The model under review builds one solid part; all positions refer to its coordinate system, in mm. Face numbers are marked on the shaded views. A direction names the side the tool comes from. Round coordinates to 2 decimals unless told otherwise and drop trailing zeros. Order: outer loops, then holes, each group sorted by start corner. A loop starts at its lowest first (then second) coordinate and runs counter-clockwise, first axis right, second up.
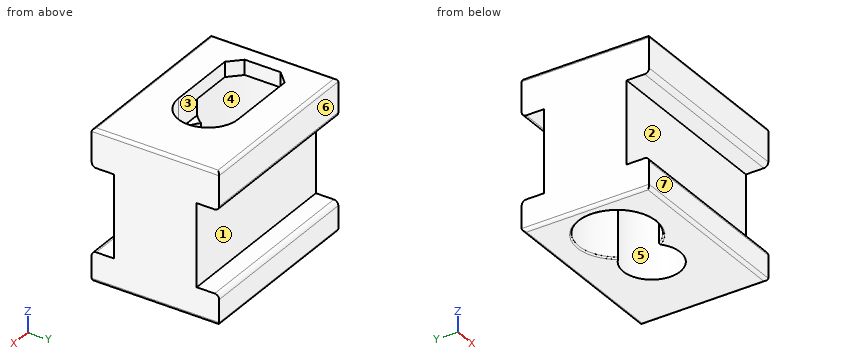
from build123d import *

# Parameters (mm, degrees)
ESQUISSE1_W             = 120
ESQUISSE1_H             = 85.2
BOSS_EXTRU_1_DEPTH      = 100
ESQUISSE2_W             = 55
ESQUISSE2_H             = 15
ENL_V_MAT_EXTRU_1_DEPTH = 121
CONG_1_R                = 3
CONG_2_R                = 2
CONG_3_R                = 2
ESQUISSE3_R             = 25.5
ENL_V_MAT_EXTRU_2_DEPTH = 90
CONG_4_R                = 1
ENL_V_MAT_EXTRU_3_DEPTH = 20.7
ESQUISSE6_R             = 19
ENL_V_MAT_EXTRU_5_DEPTH = 85


with BuildPart() as part:
    # Esquisse1 → Boss.-Extru.1 (new body)
    with BuildSketch(Plane.XY):
        Rectangle(ESQUISSE1_W, ESQUISSE1_H)
    extrude(amount=BOSS_EXTRU_1_DEPTH)

    # Esquisse2 → Enlèv. mat.-Extru.1 (cut, through all)
    with BuildSketch(Plane.ZY.offset(60)):
        with Locations((47.5, 35.1)):
            Rectangle(ESQUISSE2_W, ESQUISSE2_H)
        with Locations((47.5, -35.1)):
            Rectangle(ESQUISSE2_W, ESQUISSE2_H)
    extrude(amount=-ENL_V_MAT_EXTRU_1_DEPTH, mode=Mode.SUBTRACT)

    # Congé1
    cong_1_edges = [part.edges().sort_by_distance(p)[0] for p in [
        (0, 42.6, 75),
        (0, 42.6, 20),
        (0, -42.6, 20),
        (0, -42.6, 75),
    ]]
    fillet(cong_1_edges, radius=CONG_1_R)

    # Congé2
    cong_2_edges = [part.edges().sort_by_distance(p)[0] for p in [
        (0, -42.6, 0),
        (-60, 0, 0),
        (0, 42.6, 0),
        (60, 0, 0),
    ]]
    fillet(cong_2_edges, radius=CONG_2_R)

    # Congé3
    cong_3_edges = [part.edges().sort_by_distance(p)[0] for p in [
        (-60, 0, 100),
        (0, -42.6, 100),
        (60, 0, 100),
        (0, 42.6, 100),
    ]]
    fillet(cong_3_edges, radius=CONG_3_R)

    # Esquisse3 → Enlèv. mat.-Extru.2 (cut)
    with BuildSketch(Plane(origin=(0, 0, 0), x_dir=(-1, 0, 0), z_dir=(0, 0, -1))):
        with Locations((28, 0)):
            Circle(ESQUISSE3_R)
    extrude(amount=-ENL_V_MAT_EXTRU_2_DEPTH, mode=Mode.SUBTRACT)

    # Congé4
    cong_4_edges = [part.edges().sort_by_distance(p)[0] for p in [
        (-2.5, 0, 0),
    ]]
    fillet(cong_4_edges, radius=CONG_4_R)

    # Esquisse5 → Enlèv. mat.-Extru.3 (cut)
    with BuildSketch(Plane.XY.offset(100)):
        with BuildLine():
            Line((-48, 0), (-48, 12))
            Line((-48, 12), (-40, 20))
            Line((-40, 20), (-28, 20))
            Line((-28, 20), (6.8, 20))
            ThreePointArc((6.8, 20), (26.8, 0), (6.8, -20))
            Line((6.8, -20), (-28, -20))
            Line((-28, -20), (-40, -20))
            Line((-40, -20), (-48, -12))
            Line((-48, -12), (-48, 0))
        make_face()
    extrude(amount=-ENL_V_MAT_EXTRU_3_DEPTH, mode=Mode.SUBTRACT)

    # Esquisse6 → Enlèv. mat.-Extru.5 (cut)
    with BuildSketch(Plane.XY.offset(79.3)):
        with Locations((6.8, 0)):
            Circle(ESQUISSE6_R)
    extrude(amount=-ENL_V_MAT_EXTRU_5_DEPTH, mode=Mode.SUBTRACT)


solid = part.part
(1) To check wall thickness, follow L1, parallel to Y at x = -27, z = 5; L2, parallel to X at y = 0, z = 57; L3, parallel to Y at x = -11, z = 22. State the ranges of each line that lie inside material, in increasing order.
(2) We need section A-A (y = 34). Give the boundary of the cut face in (x, z).
(3) Tool access review of the marked faces 1, 2, 3 and 4: name each direction out of +Z, -Z, +X, -X, +Y, -Y from which nothing blocks a thin tool from reaching the whole face with its end or side.
(4) Clearance check with flat-ended pins moving along their axes: P1, Ø6, axis at x = 23, y = 9, coming from the +Z side; P2, Ø4, axis at x = 18, z = 23.5, coming from the -Y side; P3, Ø16.5, axis at x = -23, z = 60.5, coming from the +Y side. State where each tip first meets the part, or that it passes through.
(5) We need section B-B (z = 83). Give the boundary of the cut face in (x, y).
(6) The part is to be moulded in two halves that separate along Y. For the marked faces 5, 6 and 7, say which applies: pulls with the +Y half, pulls with the -Y half, needs draft (parallel to the pull), parting line crosses it, or undercut.
(7) We need section D-D (y = 0). Give the boundary of the cut face in (x, z).
Verdict:
1. L1: y = -42.6 to -25.48, 25.48 to 42.6
1. L2: x = -60 to -53.5, 25.8 to 60
1. L3: y = -27.6 to -19.01, 19.01 to 27.6
2. outline: (-60, 2) arc R2 ccw to (-58, 0) - (58, 0) arc R2 ccw to (60, 2) - (60, 20) - (-60, 20) - close; (-60, 75) - (60, 75) - (60, 98) arc R2 ccw to (58, 100) - (-58, 100) arc R2 ccw to (-60, 98) - close
3. face 1: +X, -X, +Y
3. face 2: +X, -X, -Y
3. face 3: +Z
3. face 4: -Z
4. P1: stops at z = 100
4. P2: stops at y = -27.6
4. P3: stops at y = 27.6
5. outline: (-60, -42.6) - (60, -42.6) - (60, 42.6) - (-60, 42.6) - close; hole (-12.18, -20) - (6.8, -20) arc R20 ccw to (6.8, 20) - (-12.18, 20) arc R25.5 ccw (long way) to start
6. face 5: undercut
6. face 6: pulls with the +Y half
6. face 7: pulls with the -Y half
7. outline: (-60, 2) arc R2 ccw to (-58, 0) - (-54.5, 0) arc R1 ccw to (-53.5, 1) - (-53.5, 90) - (-48, 90) - (-48, 100) - (-58, 100) arc R2 ccw to (-60, 98) - close; (25.8, 0) - (58, 0) arc R2 ccw to (60, 2) - (60, 98) arc R2 ccw to (58, 100) - (26.8, 100) - (26.8, 79.3) - (25.8, 79.3) - close
